```python
from build123d import *

# Parameters (mm, degrees)
PAD_DEPTH       = 6
FILLET_R        = 5.99
SKETCH001_R     = 8
POCKET_DEPTH    = 2.5
SKETCH002_R     = 8
POCKET001_DEPTH = 4
SKETCH003_R     = 8
POCKET002_DEPTH = 4
SKETCH004_R     = 3
POCKET003_DEPTH = 4
SKETCH005_R     = 2
PAD001_DEPTH    = 5


with BuildPart() as part:
    # Sketch → Pad (new body, symmetric)
    with BuildSketch(Plane.XY):
        with BuildLine():
            ThreePointArc((0, 7.5), (-7.5, 0), (0, -7.5))
            Line((0, -7.5), (25, -7.5))
            ThreePointArc((25, -7.5), (32.5, 0), (25, 7.5))
            Line((25, 7.5), (0, 7.5))
        make_face()
    extrude(amount=PAD_DEPTH, both=True)

    # Fillet
    fillet_edges = [part.edges().sort_by_distance(p)[0] for p in [
        (-7.5, 0, 6),
        (12.5, -7.5, 6),
        (12.5, 7.5, 6),
        (32.5, 0, 6),
        (12.5, -7.5, -6),
        (-7.5, 0, -6),
        (32.5, 0, -6),
        (12.5, 7.5, -6),
    ]]
    fillet(fillet_edges, radius=FILLET_R)

    # Sketch001 → Pocket (cut, symmetric)
    with BuildSketch(Plane.XY):
        Circle(SKETCH001_R)
    extrude(amount=POCKET_DEPTH, both=True, mode=Mode.SUBTRACT)

    # Sketch002 → Pocket001 (cut)
    with BuildSketch(Plane.XY.offset(2)):
        with Locations((25, 0)):
            Circle(SKETCH002_R)
    extrude(amount=POCKET001_DEPTH, mode=Mode.SUBTRACT)

    # Sketch003 → Pocket002 (cut)
    with BuildSketch(Plane.XY.offset(-2)):
        with Locations((25, 0)):
            Circle(SKETCH003_R)
    extrude(amount=-POCKET002_DEPTH, mode=Mode.SUBTRACT)

    # Sketch004 (on Face17 of Pocket002) → Pocket003 (cut)
    with BuildSketch(Plane.XY.offset(2)):
        with Locations((25, 0)):
            Circle(SKETCH004_R)
    extrude(amount=-POCKET003_DEPTH, mode=Mode.SUBTRACT)

    # Sketch005 (on Face6 of Pocket003) → Pad001 (join)
    with BuildSketch(Plane.XY.offset(-2.5)):
        Circle(SKETCH005_R)
    extrude(amount=PAD001_DEPTH)


solid = part.part
```
Here's how the part is built. I have some questions about the finished solid (model axes, mm). A direction names the side the tool comes from. Round coordinates to 2 decimals unless told otherwise and drop trailing zeros.
Q1. Which directions (+Z, -Z, +X, -X, +Y, -Y) give clear straight access to the entire face, cutting with the end or side of a thin tool? Please do faces 4 (the flat face through (24, 3, 2)), 5 (the flat face through (2, -1, 2.5)), 6 (the cylindrical face through (17, 0, -4)), 7 (the cylindrical face through (9.55, 5.79, -4.2)).
Q2. Will these pins go through, and if not, where does the flat tip stop? P1, Ø7, axis at x = 21, y = 1, coming from the -Z side; P2, Ø1.5, axis at x = 1, z = -3.5, coming from the -Y side; P3, Ø1.5, axis at x = 2, y = 5.5, coming from the +Z side; P4, Ø4, axis at x = 10.5, z = -2, coming from the -Y side.
Q3. Please list where these lines run through material, in increasing order: probe 1 along Y at (x, z) = (25, -0.3); probe 2 along Z at (x, y) = (7, -1.5); probe 3 along X at (y, z) = (0.5, 0).
Q4. If we mould it in two halves opening along X, with no side actions, what happens to faces 1 (the cylindrical face through (9.9, -5.79, -4.2)), 2 (the cylindrical face through (22, 0, 0)), 3 (the cylindrical face through (17, 0, 4))? For each: +X half, -X half, draft (parallel to the pull), parting line (faces both ways), or undercut.
Q5. If we section it at A-A on y = 0: Give the number of separate pieces and of enclosed holes in the cut face, plus the area to 3 significant figures.
Answer below:
1. face 4: +Z, +X
1. face 5: none
1. face 6: -Z, +X
1. face 7: -Z, +X, -X, +Y
2. P1: stops at z = -2
2. P2: stops at y = -6.84
2. P3: stops at z = 5.05
2. P4: stops at y = -7.5
3. probe 1: y = -7.49 to -3, 3 to 7.49
3. probe 2: z = -6 to -2.5, 2.5 to 6
3. probe 3: x = -1.94 to 1.94, 7.98 to 22.04, 27.96 to 32.48
4. face 1: draft
4. face 2: undercut
4. face 3: +X half
5. separate pieces: 2
5. enclosed holes: 1
5. area: 260 mm2
